Read the model definition and answer for the solid it produces. Units are mm, in the model's axes. Coordinates: 2 decimals unless noted, no trailing zeros. Order: outer loops, then holes, each group sorted by start corner. A loop starts at its lowest first (then second) coordinate and runs counter-clockwise, first axis right, second up. Notation, with made-up numbers: (-6.75, 74.5) - (42.25, 74.5) arc R22 ccw to (42.25, 88.5) - close; hole circle Ø6 at (38, 67). An arc over 180 degrees is marked (long way). Use one line per item in the form item = value.
Autodesk Inventor part; units mm, degrees
ref_plane "YZ Plane" through (0, 0, 0) normal (1, 0, 0) x (0, 1, 0)
ref_plane "XZ Plane" through (0, 0, 0) normal (0, 1, 0) x (-1, 0, 0)
ref_plane "XY Plane" through (0, 0, 0) normal (0, 0, 1) x (1, 0, 0)
sketch "Sketch1" plane through (0, 0, 0) normal (1, 0, 0) x (0, 1, 0)
  circle A0 centre (0, 0) radius 38.1 construction
  line L0 (27.94, -25.903) -> (27.94, -76.2) construction
  line L1 (27.94, -76.2) -> (-27.94, -76.2) construction
  line L2 (-27.94, -76.2) -> (-27.94, -25.903) construction
  line L3 (-30.1625, -17.4625) -> (30.1625, -17.4625) construction
  line L4 (30.1625, -17.4625) -> (30.1625, 17.4625) construction
  line L5 (30.1625, 17.4625) -> (-30.1625, 17.4625) construction
  line L6 (-30.1625, 17.4625) -> (-30.1625, -17.4625) construction
  line L7 (-30.1625, -17.4625) -> (30.1625, 17.4625) construction
  line L8 (30.1625, -17.4625) -> (-30.1625, 17.4625) construction
  circle A1 centre (30.1625, 17.4625) radius 2.5527 construction
  circle A2 centre (30.1625, -17.4625) radius 2.5527 construction
  circle A3 centre (-30.1625, -17.4625) radius 2.5527 construction
  circle A4 centre (-30.1625, 17.4625) radius 2.5527 construction
  point P0 (0, -76.2)
  dimension "d0" = 76.2
  dimension "d1" = 55.88
  dimension "d2" = 76.2
  dimension "d3" = 60.325
  dimension "d4" = 34.925
  dimension "d5" = 5.1054
  dimension "d6" = 5.1054
  dimension "d7" = 5.1054
  dimension "d8" = 5.1054
sketch "Sketch2" plane through (0, 0, 0) normal (1, 0, 0) x (0, 1, 0)
  line L0 (-30.1625, -17.4625) -> (30.1625, -17.4625) construction
  circle A0 centre (30.1625, -17.4625) radius 2.5527 construction
  circle A1 centre (-30.1625, -17.4625) radius 2.5527 construction
  line L1 (-30.1625, 17.4625) -> (-30.1625, -17.4625) construction
  circle A2 centre (-30.1625, 17.4625) radius 2.5527 construction
  line L2 (30.1625, -17.4625) -> (30.1625, 17.4625) construction
  line L3 (30.1625, -17.4625) -> (-30.1625, 17.4625) construction
  line L4 (30.1625, 17.4625) -> (-30.1625, 17.4625) construction
  line L5 (-30.1625, -17.4625) -> (30.1625, 17.4625) construction
  circle A3 centre (30.1625, 17.4625) radius 2.5527 construction
  circle A4 centre (0, 0) radius 38.1 construction
  line L6 (27.94, -25.903) -> (27.94, -76.2) construction
  line L7 (27.94, -76.2) -> (-27.94, -76.2) construction
  line L8 (-27.94, -76.2) -> (-27.94, -25.903) construction
  circle A5 centre (53.34, 0) radius 12.7 construction
  circle A6 centre (46.99, -56.6939) radius 14.2875
  circle A7 centre (46.99, -56.6939) radius 30.5054 construction
  circle A8 centre (53.34, 0) radius 9.525
  circle A9 centre (53.34, 0) radius 19.05 construction
  circle A10 centre (46.99, -56.6939) radius 20.6375 construction
  circle A11 centre (30.1625, 17.4625) radius 8.9027 construction
  circle A12 centre (30.1625, -17.4625) radius 8.9027 construction
  circle A13 centre (-30.1625, -17.4625) radius 8.9027 construction
  circle A14 centre (-30.1625, 17.4625) radius 8.9027 construction
  line L9 (58.7594, 18.2629) -> (32.6952, 25.9973)
  line L10 (30.1625, 26.3652) -> (-30.1625, 26.3652)
  line L11 (-39.0652, 17.4625) -> (-39.0652, -17.4625)
  arc A15 (72.3606, 1.0578) -> (58.7594, 18.2629) centre (53.34, 0) ccw
  arc A16 (32.6952, 25.9973) -> (30.1625, 26.3652) centre (30.1625, 17.4625) ccw
  arc A17 (-30.1625, 26.3652) -> (-39.0652, 17.4625) centre (-30.1625, 17.4625) ccw
  arc A18 (-39.0652, -17.4625) -> (-31.5677, -26.2536) centre (-30.1625, -17.4625) ccw
  circle A19 centre (46.99, -56.6939) radius 23.8125 construction
  circle A20 centre (35.0838, -36.0717) radius 4.7625 construction
  circle A21 centre (35.0838, -77.3161) radius 4.7625 construction
  circle A22 centre (70.8025, -56.6939) radius 4.7625 construction
  line L12 (72.3606, 1.0578) -> (75.5577, -56.4294)
  arc A23 (73.9775, -60.2437) -> (75.5577, -56.4294) centre (70.8025, -56.6939) ccw
  arc A24 (30.4163, -78.263) -> (36.5704, -81.8406) centre (35.0838, -77.3161) ccw
  arc A25 (30.4163, -78.263) -> (-31.5677, -26.2536) centre (-43.9964, -104.0065) ccw
  line L13 (73.9775, -60.2437) -> (60.7483, -72.0762)
  line L14 (53.4323, -76.3001) -> (36.5704, -81.8406)
  arc A26 (53.4323, -76.3001) -> (60.7483, -72.0762) centre (46.99, -56.6939) ccw
  point P0 (0, -76.2)
  point P1 (64.3385, -6.35)
  point P2 (64.3385, 6.35)
  point P3 (53.34, 12.7)
  point P4 (42.3415, 6.35)
  point P5 (42.3415, -6.35)
  point P6 (53.34, -12.7)
  dimension "d9" = 25.4
  dimension "d10" = 25.4
  dimension "d11" = 76.2
  dimension "d14" = 360
  dimension "d16" = 28.575
  dimension "d17" = 57.0484
  dimension "d18" = 19.05
  dimension "d19" = 61.0108
  dimension "d20" = 19.05
  dimension "d21" = 6.35
  dimension "d22" = 6.35
  dimension "d23" = 6.35
  dimension "d40" = 9.525
  dimension "d43" = 360
  dimension "d45" = 9.525
  dimension "d46" = 9.525
  dimension "d47" = 9.525
  dimension "d48" = 78.74
extrude "Extrusion1" add sketch "Sketch2" along normal blind 6.35
hole "Motor Mount Holes" at (0, -30.1625, -17.4625) at (0, 30.1625, -17.4625) at (0, -30.1625, 17.4625) at (0, 30.1625, 17.4625) at (0, 0, -76.2) at (0, 64.3385, -6.35) at (0, 64.3385, 6.35) at (0, 53.34, 12.7) at (0, 42.3415, 6.35) at (0, 42.3415, -6.35) at (0, 53.34, -12.7) direction (1, 0, 0) diameter 4.9784 end through all
hole "Hole3" at (0, 70.8025, -56.6939) at (0, 35.0838, -36.0717) at (0, 35.0838, -77.3161) direction (1, 0, 0) diameter 4.9784 end through all
properties part number "EL2-A-011" material "Aluminum 6061"
(1) Section D-D, the plane z = 12.7 is taken. Write down the section's boundary in (x, y), then the cut area to 3 significant figures.
Answer list:
outline = (0, -39.07) - (6.35, -39.07) - (6.35, 50.85) - (0, 50.85) - close; (0, 55.83) - (6.35, 55.83) - (6.35, 67.54) - (0, 67.54) - close
area = 645 mm2
(2) Given pin 1 Ø1.5 at (x, z) = (5.5, -49) entering from +Y; pin 2 Ø2 at (x, y) = (5.5, 5) entering from -Z, each flat-ended and moving along its own axis, determine where each tip first touches the part or whether it passes through.
Answer list:
pin_1 = 75.19
pin_2 = -43.18
(3) Section C-C, the plane x = 5.25 is taken. State how many separate pieces and enclosed holes the cut face has, then the cut area to 3 significant figures.
Answer list:
separate_pieces = 1
enclosed_holes = 15
area = 7,520 mm2
(4) Straight lines are drawn through the part: L1, parallel to Y at x = 4, z = 6.35; L2, parallel to Z at x = 3, y = 46.99; L3, parallel to Y at x = 1.75, z = -38. For each, find the intervals that lie inside material, in ascending order.
Answer list:
L1 = -39.07 to 39.85, 44.83 to 46.24, 60.44 to 61.85, 66.83 to 71.3
L2 = -78.42 to -70.98, -42.41 to -7.1, 7.1 to 21.76
L3 = -1.06 to 33.51, 36.66 to 74.53
(5) Section B-B, the plane y = 46.99 is taken. Write down the section's boundary in (x, z), then the cut area to 3 significant figures.
Answer list:
outline = (0, -78.42) - (6.35, -78.42) - (6.35, -70.98) - (0, -70.98) - close; (0, -42.41) - (6.35, -42.41) - (6.35, -7.1) - (0, -7.1) - close; (0, 7.1) - (6.35, 7.1) - (6.35, 21.76) - (0, 21.76) - close
area = 364 mm2
(6) Section A-A, the plane z = -6.35 is taken. Write down the section's boundary in (x, y).
Answer list:
outline = (0, -39.07) - (6.35, -39.07) - (6.35, 39.85) - (0, 39.85) - close; (0, 44.83) - (6.35, 44.83) - (6.35, 46.24) - (0, 46.24) - close; (0, 60.44) - (6.35, 60.44) - (6.35, 61.85) - (0, 61.85) - close; (0, 66.83) - (6.35, 66.83) - (6.35, 72.77) - (0, 72.77) - close
(7) The mould has two halves that part along Y. Classify faces 1 (the cylindrical face through (3.219, 39.873, -6.674)), 2 (the cylindrical face through (3.13, 32.74, -81.46)), 3 (the cylindrical face through (3.131, 68.182, 11.942)), 4 (the cylindrical face through (3.22, 50.87, 12.38)): +Y half, -Y half, draft (parallel to the pull), parting line (faces both ways), or undercut.
Answer list:
face_1 = undercut
face_2 = parting line
face_3 = +Y half
face_4 = undercut
